Here's how the part is built. I have some questions about the finished solid (model axes, mm). A direction names the side the tool comes from. Round coordinates to 2 decimals unless told otherwise and drop trailing zeros. Loops run counter-clockwise (first coordinate to the right, second up) from the corner with the lowest first, then second, coordinate; pieces in that order, holes last. Notation, with made-up numbers: M 47.25,80.25 L 53.25,80.25 A24 cw 53.25,115.25 Z; hole C 69.5,72 d2. An arc over 180 degrees is marked long. Use a Markdown table: item, result.
from build123d import *

# Parameters (mm, degrees)
SKETCH1_W           = 1905
SKETCH1_H           = 800.1
BOSS_EXTRUDE1_DEPTH = 76.2
BOSS_EXTRUDE2_START = 457.2
SKETCH2_W           = 1905
SKETCH2_H           = 800.1
BOSS_EXTRUDE2_DEPTH = 76.2
SKETCH3_W           = 127
SKETCH3_H           = 127
BOSS_EXTRUDE3_DEPTH = 990.6
SKETCH4_R           = 177.8
CUT_EXTRUDE1_DEPTH  = 76.2
SKETCH5_W           = 406.4
SKETCH5_H           = 406.4
CONTROL_BOX_DEPTH   = 127
SKETCH6_W           = 304.8
SKETCH6_H           = 304.8
SPECTROMETER_DEPTH  = 127


with BuildPart() as part:
    # Sketch1 → Boss-Extrude1 (new body)
    with BuildSketch(Plane(origin=(0, 0, 0), x_dir=(1, 0, 0), z_dir=(0, 1, 0))):
        Rectangle(SKETCH1_W, SKETCH1_H)
    extrude(amount=BOSS_EXTRUDE1_DEPTH)



with BuildPart() as body_2:
    # Sketch2 → Boss-Extrude2 (new body)
    with BuildSketch(Plane.XZ.offset(-76.2).offset(BOSS_EXTRUDE2_START)):
        Rectangle(SKETCH2_W, SKETCH2_H)
    extrude(amount=BOSS_EXTRUDE2_DEPTH)


with BuildPart() as part_1:
    add(part.part)

    add(body_2.part)  # Boss-Extrude3 merges body 2
    # Sketch3 → Boss-Extrude3 (add)
    with BuildSketch(Plane(origin=(0, 76.2, 0), x_dir=(1, 0, 0), z_dir=(0, 1, 0))):
        with Locations((-889, -336.55)):
            Rectangle(SKETCH3_W, SKETCH3_H)
        with Locations((889, 336.55)):
            Rectangle(SKETCH3_W, SKETCH3_H)
        with Locations((-889, 336.55)):
            Rectangle(SKETCH3_W, SKETCH3_H)
        with Locations((889, -336.55)):
            Rectangle(SKETCH3_W, SKETCH3_H)
    extrude(amount=-BOSS_EXTRUDE3_DEPTH)

    # Sketch4 → Cut-Extrude1 (cut)
    with BuildSketch(Plane(origin=(0, 76.2, 0), x_dir=(1, 0, 0), z_dir=(0, 1, 0))):
        with Locations((88.9, 0)):
            Circle(SKETCH4_R)
    extrude(amount=-CUT_EXTRUDE1_DEPTH, mode=Mode.SUBTRACT)

    # Sketch5 → Control Box (add)
    with BuildSketch(Plane(origin=(0, -381, 0), x_dir=(1, 0, 0), z_dir=(0, 1, 0))):
        with Locations((152.685371452, 1.975779164)):
            Rectangle(SKETCH5_W, SKETCH5_H)
    extrude(amount=CONTROL_BOX_DEPTH)

    # Sketch6 → Spectrometer (add)
    with BuildSketch(Plane(origin=(0, -381, 0), x_dir=(1, 0, 0), z_dir=(0, 1, 0))):
        with Locations((-673.1, -6.35)):
            Rectangle(SKETCH6_W, SKETCH6_H)
    extrude(amount=SPECTROMETER_DEPTH)


solid = part_1.part
1. Imagine slicing it at A-A, the plane y = -626.5. Write out the boundary of the cut face in (x, z).
Answer sheet:
| item | result |
|---|---|
| outline | M -952.5,-400.05 L -825.5,-400.05 L -825.5,-273.05 L -952.5,-273.05 Z; M -952.5,273.05 L -825.5,273.05 L -825.5,400.05 L -952.5,400.05 Z; M 825.5,-400.05 L 952.5,-400.05 L 952.5,-273.05 L 825.5,-273.05 Z; M 825.5,273.05 L 952.5,273.05 L 952.5,400.05 L 825.5,400.05 Z |
2. Imagine slicing it at C-C, the plane z = 0. Write out the boundary of the cut face in (x, y), then the cut area to 3 significant figures.
Answer sheet:
| item | result |
|---|---|
| outline | M -952.5,-457.2 L 952.5,-457.2 L 952.5,-381 L 355.89,-381 L 355.89,-254 L -50.51,-254 L -50.51,-381 L -520.7,-381 L -520.7,-254 L -825.5,-254 L -825.5,-381 L -952.5,-381 Z; M -952.5,0 L -88.9,0 L -88.9,76.2 L -952.5,76.2 Z; M 266.7,0 L 952.5,0 L 952.5,76.2 L 266.7,76.2 Z |
| area | 354,000 mm2 |
3. Which directions (+Z, -Z, +X, -X, +Y, -Y) give clear straight access to the entire face, cutting with the end or side of a thin tool? Please do faces 4 (the face through (-225, -381, 6)), 5 (the face through (150, -318, 201.224)), 6 (the face through (-825.5, -318, 8)), 7 (the face through (-675, -254, 4)), 8 (the face through (-825.5, -188, -336)).
Answer sheet:
| item | result |
|---|---|
| face 4 | none |
| face 5 | +Z, +X, -X |
| face 6 | -X |
| face 7 | +Z, -Z, +X, -X |
| face 8 | -Z |
4. Imagine slicing it at D-D, the plane y = -283.5. Write out the boundary of the cut face in (x, z).
Answer sheet:
| item | result |
|---|---|
| outline | M -952.5,-400.05 L -825.5,-400.05 L -825.5,-273.05 L -952.5,-273.05 Z; M -952.5,273.05 L -825.5,273.05 L -825.5,400.05 L -952.5,400.05 Z; M -825.5,-146.05 L -520.7,-146.05 L -520.7,158.75 L -825.5,158.75 Z; M -50.51,-205.18 L 355.89,-205.18 L 355.89,201.22 L -50.51,201.22 Z; M 825.5,-400.05 L 952.5,-400.05 L 952.5,-273.05 L 825.5,-273.05 Z; M 825.5,273.05 L 952.5,273.05 L 952.5,400.05 L 825.5,400.05 Z |
5. I need wall thicknesses on probe 1 along X at (y, z) = (-723.5, 367); probe 2 along Y at (x, z) = (-40, 202); probe 3 along X at (y, z) = (58.5, 0). Which ranges of each line are inside material? Lowest first, please. Write a range as from..to.
Answer sheet:
| item | result |
|---|---|
| probe 1 | -952.5..-825.5, 825.5..952.5 |
| probe 2 | -457.2..-381, 0..76.2 |
| probe 3 | -952.5..-88.9, 266.7..952.5 |
6. Imagine slicing it at B-B, the plane x = 592.5. Write out the boundary of the cut face in (y, z).
Answer sheet:
| item | result |
|---|---|
| outline | M -457.2,-400.05 L -381,-400.05 L -381,400.05 L -457.2,400.05 Z; M 0,-400.05 L 76.2,-400.05 L 76.2,400.05 L 0,400.05 Z |
7. For pin 1 Ø5 at (y, z) = (-322, -3) entering from -X; pin 2 Ø4 at (x, z) = (-683.5, -3.5) entering from -Y, each with a flat end and sliding along its axis, tell me the tip position at first contact or that it passes through.
Answer sheet:
| item | result |
|---|---|
| pin 1 | x = -825.5 |
| pin 2 | y = -457.2 |
8. We'd pull the mould along Y, two halves only. Please class faces 1 (the face through (-88.728, 38.633, -7.818)), 2 (the face through (-890, -188, -273.05)), 3 (the face through (-13, 76.2, -183)): +Y half, -Y half, draft (parallel to the pull), parting line (faces both ways), or undercut.
Answer sheet:
| item | result |
|---|---|
| face 1 | draft |
| face 2 | undercut |
| face 3 | +Y half |
